Work out the finished part from the listing and answer in its coordinate system (mm). Round coordinates to 2 decimals unless told otherwise and drop trailing zeros. Order: outer loops, then holes, each group sorted by start corner. A loop starts at its lowest first (then second) coordinate and runs counter-clockwise, first axis right, second up. Notation, with made-up numbers: (33.5, 87.25) - (60.5, 87.25) arc R34 ccw to (60.5, 124.25) - close; hole circle Ø5 at (62, 10). An arc over 180 degrees is marked (long way). Put each result on its own line as item: value.
Autodesk Inventor part; units mm, degrees
ref_plane "YZ Plane" through (0, 0, 0) normal (1, 0, 0) x (0, 1, 0)
ref_plane "XZ Plane" through (0, 0, 0) normal (0, 1, 0) x (-1, 0, 0)
ref_plane "XY Plane" through (0, 0, 0) normal (0, 0, 1) x (1, 0, 0)
sketch "Sketch2" plane through (0, 0, 0) normal (0, 1, 0) x (-1, 0, 0)
  line L0 (-89, 99) -> (89, 99)
  line L1 (89, 99) -> (89, -99)
  line L2 (89, -99) -> (-89, -99)
  line L3 (-89, -99) -> (-89, 99)
  line L4 (-89, 99) -> (89, -99) construction
  line L5 (89, 99) -> (-89, -99) construction
  line L6 (-89, 99) -> (89, 99)
  line L7 (89, 99) -> (89, -81)
  line L8 (89, -81) -> (-89, -81)
  line L9 (-89, -81) -> (-89, 99)
  line L10 (-4.5, 99) -> (-89, 99)
  line L11 (-89, 99) -> (-89, 43)
  line L12 (-89, 43) -> (-4.5, 43)
  line L13 (-4.5, 43) -> (-4.5, 99)
  line L14 (4.5, 99) -> (89, 99)
  line L15 (89, 99) -> (89, 43)
  line L16 (89, 43) -> (4.5, 43)
  line L17 (4.5, 43) -> (4.5, 99)
  line L18 (22.5, 77.5) -> (22.5, 66.5)
  line L19 (16.5, 66.5) -> (16.5, 77.5)
  line L20 (-22.5, 66.5) -> (-22.5, 77.5)
  line L21 (-16.5, 77.5) -> (-16.5, 66.5)
  line L22 (-22.5, 99) -> (-16.5, 99)
  line L23 (-16.5, 99) -> (-16.5, 43)
  line L24 (-16.5, 43) -> (-22.5, 43)
  line L25 (-22.5, 43) -> (-22.5, 99)
  line L26 (16.5, 99) -> (22.5, 99)
  line L27 (22.5, 99) -> (22.5, 43)
  line L28 (22.5, 43) -> (16.5, 43)
  line L29 (16.5, 43) -> (16.5, 99)
  line L30 (-89, 99) -> (89, 99)
  line L31 (89, 99) -> (89, 98)
  line L32 (89, 98) -> (-89, 98)
  line L33 (-89, 98) -> (-89, 99)
  line L34 (89, -81) -> (74, -81)
  line L35 (74, -81) -> (74, -65)
  line L36 (74, -65) -> (89, -65)
  line L37 (89, -65) -> (89, -81)
  line L38 (-89, -81) -> (-74, -81)
  line L39 (-74, -81) -> (-74, -65)
  line L40 (-74, -65) -> (-89, -65)
  line L41 (-89, -65) -> (-89, -81)
  point P0 (0, 0)
  point P1 (4.5, 99)
  point P2 (-4.5, 99)
  point P3 (-89, 43)
  point P4 (89, 43)
  point P5 (4.5, 98)
  point P6 (-4.5, 98)
  point P7 (-16.5, 98)
  point P8 (-22.5, 98)
  point P9 (22.5, 98)
  point P10 (16.5, 98)
  dimension "d8" = 178
  dimension "d9" = 198
  dimension "d10" = 18
  dimension "d11" = 84.5
  dimension "d13" = 84.5
  dimension "d17" = 9
  dimension "d18" = 1
  dimension "d19" = 15
  dimension "d20" = 16
  dimension "d21" = 15
  dimension "d22" = 16
  dimension "d75" = 55
  dimension "d76" = 55
extrude "Extrusion2" add sketch "Sketch2" along normal blind 3 contours L32 L23 L21 L12 L25 L20 | L12 L13 L32 L17 L16 L1 L36 L35 L8 L39 L40 L3 | L32 L27 L18 L16 L29 L19
fillet "Fillet1" radius 3 6 edges at (22.5, 1.5, 43) (-22.5, 1.5, 43) (-16.5, 1.5, 43) (-4.5, 1.5, 43) (4.5, 1.5, 43) (16.5, 1.5, 43)
fillet "Fillet2" radius 3 2 edges at (74, 1.5, -65) (-74, 1.5, -65)
equation "\"d11\" = d13"
properties part number "base" material "Aluminum 6061"
1) Given pin 1 Ø1.5 at (y, z) = (2, 79) entering from -X; pin 2 Ø1.5 at (x, y) = (-44.5, 1) entering from +Z; pin 3 Ø1.5 at (x, y) = (86, 1.5) entering from -Z, each flat-ended and moving along its own axis, determine where each tip first touches the part or whether it passes through.
Findings below:
pin 1: stops at x = -22.5
pin 2: stops at z = 43
pin 3: stops at z = -65
2) A cutting plane is placed at A-A on z = 65. Write down the section's boundary in (x, y), then the cut area to 3 significant figures.
Findings below:
outline: (-22.5, 0) - (-16.5, 0) - (-16.5, 3) - (-22.5, 3) - close; (-4.5, 0) - (4.5, 0) - (4.5, 3) - (-4.5, 3) - close; (16.5, 0) - (22.5, 0) - (22.5, 3) - (16.5, 3) - close
area: 63.0 mm2
3) A cutting plane is placed at B-B on y = 2.05. Write down the section's boundary in (x, z), then the cut area to 3 significant figures.
Findings below:
outline: (-89, -65) - (-77, -65) arc R3 cw to (-74, -68) - (-74, -81) - (74, -81) - (74, -68) arc R3 cw to (77, -65) - (89, -65) - (89, 43) - (25.5, 43) arc R3 cw to (22.5, 46) - (22.5, 98) - (16.5, 98) - (16.5, 46) arc R3 cw to (13.5, 43) - (7.5, 43) arc R3 cw to (4.5, 46) - (4.5, 98) - (-4.5, 98) - (-4.5, 46) arc R3 cw to (-7.5, 43) - (-13.5, 43) arc R3 cw to (-16.5, 46) - (-16.5, 98) - (-22.5, 98) - (-22.5, 46) arc R3 cw to (-25.5, 43) - (-89, 43) - close
area: 22,800 mm2
4) A cutting plane is placed at C-C on x = -64.5. Write down the section's boundary in (y, z).
Findings below:
outline: (0, -81) - (3, -81) - (3, 43) - (0, 43) - close
5) Straight lines are drawn through the part: L1, parallel to X at y = 0.3, z = 54; L2, parallel to Z at x = -55, y = 1.25; L3, parallel to X at y = 0.8, z = 44. For each, find the intervals that lie inside material, in ascending order. Write a range as from..to.
Findings below:
L1: x = -22.5..-16.5, -4.5..4.5, 16.5..22.5
L2: z = -81..43
L3: x = -23.26..-15.74, -5.26..5.26, 15.74..23.26
